Could you check a few things on this drawing? It's one solid part, dimensions in mm from its lowest x, y, z. A direction names the side the tool comes from. Give positions to 0.01 mm unless a question says otherwise; leave off trailing zeros. Loops run counter-clockwise (first coordinate to the right, second up) from the corner with the lowest first, then second, coordinate; pieces in that order, holes last. Notation, with made-up numbers: M -23.5,33 L 34.5,33 A22 cw 34.5,45 Z; hole C 7,29.5 d2. An arc over 180 degrees is marked long. Write each question's results on one line, items separated by ' | '. Start each with the question number.
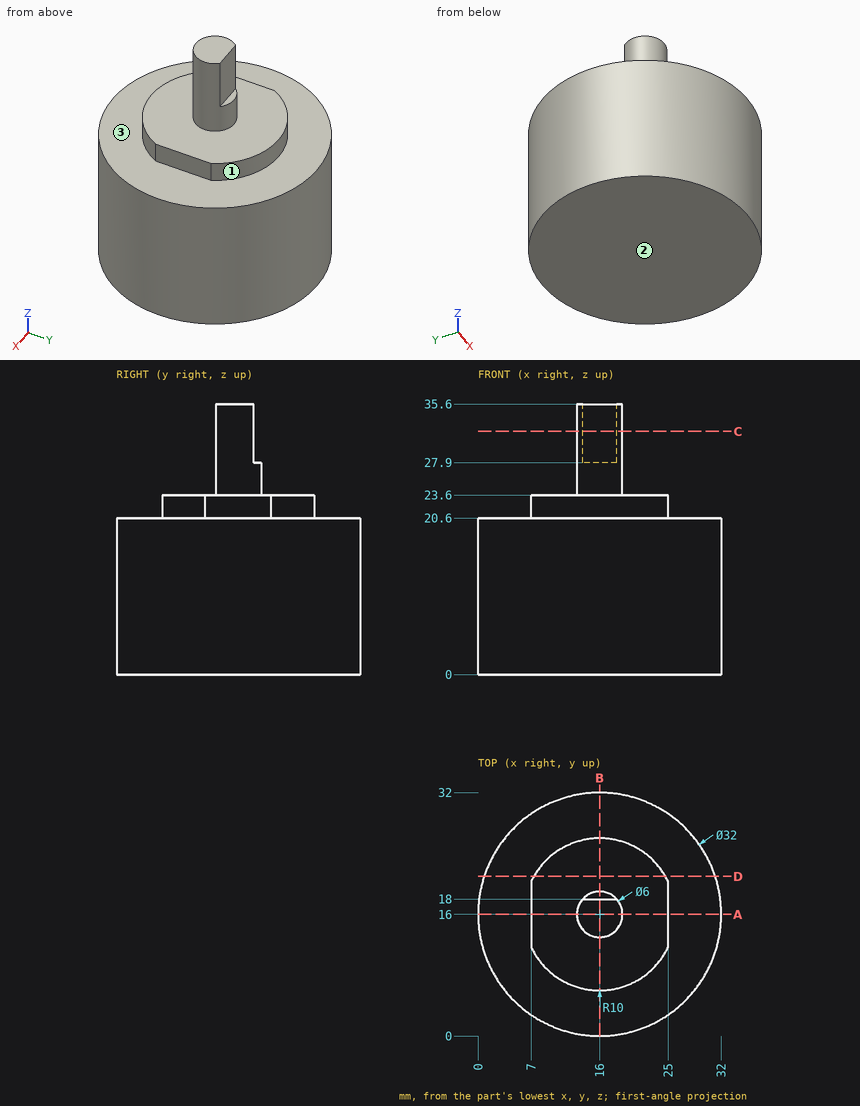
1) I'm going to push flat-ended pins straight in: P1, Ø8, axis at x = 10, y = 9.5, coming from the +Z side; P2, Ø1, axis at y = 11, z = 14, coming from the -X side; P3, Ø3.5, axis at y = 14.5, z = 22, coming from the -X side. Where does each tip first touch, or does it pass through?
2) If we section it at B-B on x = 16: Write out the boundary of the cut face in (y, z), plus the area to 4 significant figures.
3) If we section it at C-C on z = 32: Write out the boundary of the cut face in (x, y), plus the area to 3 significant figures.
4) If we section it at D-D on y = 21: Write out the boundary of the cut face in (x, z), plus the area to 3 significant figures.
5) Please list where these lines run through material, in increasing order: line 1 (Z direction, x = 15.5, y = 13); line 2 (Z direction, x = 2, y = 12); line 3 (X direction, y = 14.5, z = 25). Write a range as from..to.
6) Which directions (+Z, -Z, +X, -X, +Y, -Y) give clear straight access to the entire face, cutting with the end or side of a thin tool? Please do the marked faces 1, 2 and 3.
7) If we section it at A-A on y = 16: Write out the boundary of the cut face in (x, z), plus the area to 3 significant figures.
Calculated:
1) P1: stops at z = 23.6 | P2: stops at x = 0.65 | P3: stops at x = 0.01
2) outline: M 0,0 L 32,0 L 32,20.6 L 26,20.6 L 26,23.6 L 19,23.6 L 19,27.9 L 18,27.9 L 18,35.6 L 13,35.6 L 13,23.6 L 6,23.6 L 6,20.6 L 0,20.6 Z | area: 783.5 mm2
3) outline: M 13.76,18 A3 ccw long 18.24,18 Z | area: 25.2 mm2
4) outline: M 0.8,0 L 31.2,0 L 31.2,20.6 L 24.66,20.6 L 24.66,23.6 L 7.34,23.6 L 7.34,20.6 L 0.8,20.6 Z | area: 678 mm2
5) line 1: z = 0..23.6 | line 2: z = 0..20.6 | line 3: x = 13.4..18.6
6) face 1: +Z, +Y | face 2: -Z, +X, -X, +Y, -Y | face 3: +Z
7) outline: M 0,0 L 32,0 L 32,20.6 L 25,20.6 L 25,23.6 L 19,23.6 L 19,35.6 L 13,35.6 L 13,23.6 L 7,23.6 L 7,20.6 L 0,20.6 Z | area: 785 mm2
